```python
from build123d import *

# Parameters (mm, degrees)
SKETCH1_R                            = 49
BOSS_EXTRUDE1_DEPTH                  = 3
SKETCH2_R                            = 24.5
CUT_EXTRUDE1_DEPTH                   = 3
SKETCH3_R                            = 3.150000005
CUT_EXTRUDE2_DEPTH                   = 3
SKETCH5_W                            = 50
SKETCH5_H                            = 3
BOSS_EXTRUDE3_DEPTH                  = 10
BOSS_EXTRUDE3_DIRECTION_2_REACH      = 111.608
BOSS_EXTRUDE3_DIRECTION_2_END_RADIUS = 49
SKETCH6_W                            = 5
SKETCH6_H                            = 3
BOSS_EXTRUDE4_DEPTH                  = 4
FILLET1_R                            = 1.5
LPATTERN3_COUNT                      = 5
LPATTERN3_PITCH                      = 11.25
FILLET1_OF_LPATTERN3_R               = 1.5
CUT_EXTRUDE3_DEPTH                   = 98.231682079
CUT_EXTRUDE3_DEPTH_BACK              = 98.231682079
SKETCH7_R                            = 0.756640097


with BuildPart() as part:
    # Sketch1 → Boss-Extrude1 (new body)
    with BuildSketch(Plane.XY):
        Circle(SKETCH1_R)
    extrude(amount=BOSS_EXTRUDE1_DEPTH)

    # Sketch2 → Cut-Extrude1 (cut)
    with BuildSketch(Plane.XY.offset(3)):
        Circle(SKETCH2_R)
    extrude(amount=-CUT_EXTRUDE1_DEPTH, mode=Mode.SUBTRACT)

    # Sketch3 → Cut-Extrude2 (cut)
    with BuildSketch(Plane.XY.offset(3)):
        with Locations((16.264045876, -39.264880132)):
            Circle(SKETCH3_R)
        with Locations((39.264880132, -16.264045875)):
            Circle(SKETCH3_R)
        with Locations((39.264880132, 16.264045876)):
            Circle(SKETCH3_R)
        with Locations((16.264045876, 39.264880132)):
            Circle(SKETCH3_R)
        with Locations((-16.264045875, 39.264880132)):
            Circle(SKETCH3_R)
        with Locations((-39.264880132, 16.264045876)):
            Circle(SKETCH3_R)
        with Locations((-39.264880132, -16.264045875)):
            Circle(SKETCH3_R)
        with Locations((-16.264045875, -39.264880132)):
            Circle(SKETCH3_R)
    extrude(amount=-CUT_EXTRUDE2_DEPTH, mode=Mode.SUBTRACT)

    # Sketch5 → Boss-Extrude3 (add)
    with BuildSketch(Plane(origin=(0, 49, 0), x_dir=(1, 0, 0), z_dir=(0, 1, 0))):
        with Locations((0, -1.5)):
            Rectangle(SKETCH5_W, SKETCH5_H)
    extrude(amount=BOSS_EXTRUDE3_DEPTH)

    # Boss-Extrude3 direction 2: up to this cylinder (the profile starts outside it)
    boss_extrude3_direction_2_end = Plane(origin=(0, 0, 1.5), z_dir=(0, 0, -1)) * Cylinder(BOSS_EXTRUDE3_DIRECTION_2_END_RADIUS, 322.216, mode=Mode.PRIVATE)
    # Sketch5 → Boss-Extrude3 direction 2 (add, up to the surface)
    with BuildSketch(Plane(origin=(0, 49, 0), x_dir=(1, 0, 0), z_dir=(0, 1, 0)), mode=Mode.PRIVATE) as boss_extrude3_direction_2_sk1:
        with Locations((0, -1.5)):
            Rectangle(SKETCH5_W, SKETCH5_H)
    boss_extrude3_direction_2_tool1 = extrude(boss_extrude3_direction_2_sk1.sketch, amount=-BOSS_EXTRUDE3_DIRECTION_2_REACH, mode=Mode.PRIVATE) - boss_extrude3_direction_2_end
    add(boss_extrude3_direction_2_tool1.solids().sort_by_distance((0, 49, 1.5))[0])
    add(boss_extrude3_direction_2_tool1.solids().sort_by_distance((0, 49, 1.5))[1])

    # Sketch6 → Boss-Extrude4 (add)
    with BuildSketch(Plane(origin=(0, 59, 0), x_dir=(1, 0, 0), z_dir=(0, 1, 0))):
        with Locations((-22.5, -1.5)):
            Rectangle(SKETCH6_W, SKETCH6_H)
    boss_extrude4 = extrude(amount=BOSS_EXTRUDE4_DEPTH)

    # Fillet1
    fillet1_edges = [part.edges().sort_by_distance(p)[0] for p in [
        (-22.5, 63, 0),
        (-22.5, 63, 3),
    ]]
    fillet(fillet1_edges, radius=FILLET1_R - 0.0001)  # a hair under: the kernel refuses the full size

    # LPattern3: Boss-Extrude4 ×5
    with Locations(*[(i * LPATTERN3_PITCH, 0, 0) for i in range(1, LPATTERN3_COUNT)]):
        add(boss_extrude4)

    # Fillet1 of LPattern3
    fillet1_of_lpattern3_edges = [part.edges().sort_by_distance(p)[0] for p in [
        (-11.25, 63, 0),
        (-11.25, 63, 3),
        (0, 63, 0),
        (0, 63, 3),
        (11.25, 63, 0),
        (11.25, 63, 3),
        (22.5, 63, 0),
        (22.5, 63, 3),
    ]]
    fillet(fillet1_of_lpattern3_edges, radius=FILLET1_OF_LPATTERN3_R - 0.0001)  # a hair under: the kernel refuses the full size

    # Sketch7 → Cut-Extrude3 (cut, two sides: drawn at the far end of the back side and taken through both)
    with BuildSketch(Plane.ZY.offset(25).offset(-CUT_EXTRUDE3_DEPTH_BACK)):
        with Locations(Location((1.5, 61.5, 0), (0, 0, 180))):
            Circle(SKETCH7_R)
    extrude(amount=CUT_EXTRUDE3_DEPTH + CUT_EXTRUDE3_DEPTH_BACK, mode=Mode.SUBTRACT)


solid = part.part
```
Can you work these out from the model? Positions are in its coordinate system, mm. A direction names the side the tool comes from. Give positions to 0.01 mm unless a question says otherwise; leave off trailing zeros. Write each loop counter-clockwise with the first axis right and the second up, starting at its lowest first coordinate (ties: lowest second). Pieces come first, ordered by that corner, then holes. Notation, with made-up numbers: (12, 69) - (42, 69) arc R17 ccw to (42, 82) - close; hole circle Ø11 at (-22, 48). An arc over 180 degrees is marked (long way). Write item = value, one per line. Start each with the question number.
1. Imagine slicing it at B-B (y = 0). Please give me the cut outline in (x, z).
2. Imagine slicing it at D-D (x = -39). Please give me the cut outline in (y, z), and give its area (3 significant figures).
3. On a 3-axis mill with a long thin cutter (end or side, diameter ignored), from which of +Z, -Z, +X, -X, +Y, -Y can I reach the whole of each face in a straight line? I mean faces 5 (the face through (-2.5, 60.5, 1.5)), 6 (the face through (-18.764, 37.348, 1.521)). Say none if no direction works.
4. Imagine slicing it at A-A (x = 0). Count the separate pieces of the cut face and the enclosed holes in it, and give its area (3 significant figures).
5. Thinking about a two-plate mould opening in X: for faces 1 (the face through (36.94, 18.39, 1.52)), 2 (the face through (-17, 59, 1)), 3 (the face through (-25, 52, 2)), 4 (the face through (-1, 30, 0)), which applies, released by +X, released by -X, zero draft, split by the parting line, or undercut?
6. Please list where these lines run through material, in increasing order: line 1 (Y direction, x = -42, z = 2.8); line 2 (Y direction, x = -40, z = 1.1); line 3 (X direction, y = -19, z = 2.85).
7. For pin 1 (1.5 mm diameter, centred on y = 61, z = 1, fed in from +X); pin 2 (8 mm diameter, centred on x = 39.26, y = -16.26, fed in from -Z); pin 3 (1 mm diameter, centred on x = 16.5, z = 2.5, fed in from -Y); pin 4 (1 mm diameter, centred on y = 35, z = 1, fed in from -X), each with a flat end and sliding along its axis, tell me the tip position at first contact or that it passes through.
Worked answers:
q1.outline = (-49, 0) - (-24.5, 0) - (-24.5, 3) - (-49, 3) - close; (24.5, 0) - (49, 0) - (49, 3) - (24.5, 3) - close
q2.outline = (-29.66, 0) - (-19.4, 0) - (-19.4, 3) - (-29.66, 3) - close; (-13.13, 0) - (13.13, 0) - (13.13, 3) - (-13.13, 3) - close; (19.4, 0) - (29.66, 0) - (29.66, 3) - (19.4, 3) - close
q2.area = 140 mm2
q3.face_5 = +Z, -Z, +Y
q3.face_6 = +Z, -Z
q4.separate_pieces = 2
q4.enclosed_holes = 1
q4.area = 186 mm2
q5.face_1 = undercut
q5.face_2 = undercut
q5.face_3 = released by -X
q5.face_4 = zero draft
q6.line_1 = -25.24 to -17.83, -14.7 to 14.7, 17.83 to 25.24
q6.line_2 = -28.3 to -19.33, -13.2 to 13.2, 19.33 to 28.3
q6.line_3 = -45.17 to -40.83, -37.7 to -15.47, 15.47 to 37.7, 40.83 to 45.17
q7.pin_1 = 25
q7.pin_2 = 0
q7.pin_3 = -46.31
q7.pin_4 = -34.8
